```python
from build123d import *

# Parameters (mm, degrees)
BOSS_EXTRUDE1_DEPTH        = 1.5
SKETCH3_R                  = 2.5
SKETCH3_R_2                = 1
SKETCH3_R_3                = 2
BOSS_EXTRUDE2_DEPTH        = 3
F_4_8_4_8_DIAMETER_HOLE1_D = 4.8
SKETCH7_R                  = 4.75
SKETCH7_R_2                = 2.4
BOSS_EXTRUDE3_DEPTH        = 2.7
F_2_0MM_DOWEL_HOLE1_D      = 2
CHAMFER1_SIZE              = 1
SKETCH15_R                 = 2.38125
CUT_EXTRUDE1_DEPTH         = 126.335549626


with BuildPart() as part:
    # Sketch2 → Boss-Extrude1 (new, symmetric)
    with BuildSketch(Plane(origin=(0, 0, 0), x_dir=(1, 0, 0), z_dir=(0, 1, 0))):
        with BuildLine():
            Line((-50, -110), (50, -110))
            ThreePointArc((50, -110), (57.071067812, -107.071067812), (60, -100))
            Line((60, -100), (60, 100))
            ThreePointArc((60, 100), (57.071067812, 107.071067812), (50, 110))
            Line((50, 110), (-50, 110))
            ThreePointArc((-50, 110), (-57.071067812, 107.071067812), (-60, 100))
            Line((-60, 100), (-60, -100))
            ThreePointArc((-60, -100), (-57.071067812, -107.071067812), (-50, -110))
        make_face()
    extrude(amount=BOSS_EXTRUDE1_DEPTH, both=True)

    # Sketch3 → Boss-Extrude2 (add)
    # profile 1 of 16: a face of its own
    with BuildSketch(Plane(origin=(0, 1.5, 0), x_dir=(1, 0, 0), z_dir=(0, 1, 0))):
        with Locations(Location((41.24318761, -46.24391141, 0), (0, 0, 90))):
            Circle(SKETCH3_R)
        with Locations(Location((41.24318761, -46.24391141, 0), (0, 0, 270))):
            Circle(SKETCH3_R_2, mode=Mode.SUBTRACT)
    # profile 2 of 16: a face of its own
    with BuildSketch(Plane(origin=(0, 1.5, 0), x_dir=(1, 0, 0), z_dir=(0, 1, 0))):
        with Locations(Location((3.86368673, -46.24391141, 0), (0, 0, 90))):
            Circle(SKETCH3_R)
        with Locations(Location((3.86368673, -46.24391141, 0), (0, 0, 270))):
            Circle(SKETCH3_R_2, mode=Mode.SUBTRACT)
    # profile 3 of 16: a face of its own
    with BuildSketch(Plane(origin=(0, 1.5, 0), x_dir=(1, 0, 0), z_dir=(0, 1, 0))):
        with Locations(Location((3.86368673, -82.98571173, 0), (0, 0, 90))):
            Circle(SKETCH3_R)
        with Locations(Location((3.86368673, -82.98571173, 0), (0, 0, 270))):
            Circle(SKETCH3_R_2, mode=Mode.SUBTRACT)
    # profile 4 of 16: a face of its own
    with BuildSketch(Plane(origin=(0, 1.5, 0), x_dir=(1, 0, 0), z_dir=(0, 1, 0))):
        with Locations(Location((41.24318761, -82.98571173, 0), (0, 0, 90))):
            Circle(SKETCH3_R)
        with Locations(Location((41.24318761, -82.98571173, 0), (0, 0, 270))):
            Circle(SKETCH3_R_2, mode=Mode.SUBTRACT)
    # profile 5 of 16: a face of its own
    with BuildSketch(Plane(origin=(0, 1.5, 0), x_dir=(1, 0, 0), z_dir=(0, 1, 0))):
        with Locations(Location((-10.13631327, -24.98571173, 0), (0, 0, 90))):
            Circle(SKETCH3_R)
        with Locations(Location((-10.13631327, -24.98571173, 0), (0, 0, 270))):
            Circle(SKETCH3_R_2, mode=Mode.SUBTRACT)
    # profile 6 of 16: a face of its own
    with BuildSketch(Plane(origin=(0, 1.5, 0), x_dir=(1, 0, 0), z_dir=(0, 1, 0))):
        with Locations(Location((-10.13631327, 11.75608859, 0), (0, 0, 90))):
            Circle(SKETCH3_R)
        with Locations(Location((-10.13631327, 11.75608859, 0), (0, 0, 270))):
            Circle(SKETCH3_R_2, mode=Mode.SUBTRACT)
    # profile 7 of 16: a face of its own
    with BuildSketch(Plane(origin=(0, 1.5, 0), x_dir=(1, 0, 0), z_dir=(0, 1, 0))):
        with Locations(Location((27.24318761, 11.75608859, 0), (0, 0, 90))):
            Circle(SKETCH3_R)
        with Locations(Location((27.24318761, 11.75608859, 0), (0, 0, 270))):
            Circle(SKETCH3_R_2, mode=Mode.SUBTRACT)
    # profile 8 of 16: a face of its own
    with BuildSketch(Plane(origin=(0, 1.5, 0), x_dir=(1, 0, 0), z_dir=(0, 1, 0))):
        with Locations(Location((27.24318761, -24.98571173, 0), (0, 0, 90))):
            Circle(SKETCH3_R)
        with Locations(Location((27.24318761, -24.98571173, 0), (0, 0, 270))):
            Circle(SKETCH3_R_2, mode=Mode.SUBTRACT)
    # profile 9 of 16: a face of its own
    with BuildSketch(Plane(origin=(0, 1.5, 0), x_dir=(1, 0, 0), z_dir=(0, 1, 0))):
        with Locations(Location((-48.56, -75.45, 0), (0, 0, 90))):
            Circle(SKETCH3_R_3)
        with Locations(Location((-48.56, -75.45, 0), (0, 0, 270))):
            Circle(SKETCH3_R_2, mode=Mode.SUBTRACT)
    # profile 10 of 16: a face of its own
    with BuildSketch(Plane(origin=(0, 1.5, 0), x_dir=(1, 0, 0), z_dir=(0, 1, 0))):
        with Locations(Location((-32.54, -45.15, 0), (0, 0, 90))):
            Circle(SKETCH3_R_3)
        with Locations(Location((-32.54, -45.15, 0), (0, 0, 270))):
            Circle(SKETCH3_R_2, mode=Mode.SUBTRACT)
    # profile 11 of 16: a face of its own
    with BuildSketch(Plane(origin=(0, 1.5, 0), x_dir=(1, 0, 0), z_dir=(0, 1, 0))):
        with Locations(Location((-48.56, -21.95, 0), (0, 0, 90))):
            Circle(SKETCH3_R_3)
        with Locations(Location((-48.56, -21.95, 0), (0, 0, 270))):
            Circle(SKETCH3_R_2, mode=Mode.SUBTRACT)
    # profile 12 of 16: a face of its own
    with BuildSketch(Plane(origin=(0, 1.5, 0), x_dir=(1, 0, 0), z_dir=(0, 1, 0))):
        with Locations(Location((-32.54, 8.35, 0), (0, 0, 90))):
            Circle(SKETCH3_R_3)
        with Locations(Location((-32.54, 8.35, 0), (0, 0, 270))):
            Circle(SKETCH3_R_2, mode=Mode.SUBTRACT)
    # profile 13 of 16: a face of its own
    with BuildSketch(Plane(origin=(0, 1.5, 0), x_dir=(1, 0, 0), z_dir=(0, 1, 0))):
        with Locations(Location((-39.7, 32.2, 0), (0, 0, 90))):
            Circle(SKETCH3_R)
        with Locations(Location((-39.7, 32.2, 0), (0, 0, 270))):
            Circle(SKETCH3_R_2, mode=Mode.SUBTRACT)
    # profile 14 of 16: a face of its own
    with BuildSketch(Plane(origin=(0, 1.5, 0), x_dir=(1, 0, 0), z_dir=(0, 1, 0))):
        with Locations(Location((-38.6, 80, 0), (0, 0, 90))):
            Circle(SKETCH3_R)
        with Locations(Location((-38.6, 80, 0), (0, 0, 270))):
            Circle(SKETCH3_R_2, mode=Mode.SUBTRACT)
    # profile 15 of 16: a face of its own
    with BuildSketch(Plane(origin=(0, 1.5, 0), x_dir=(1, 0, 0), z_dir=(0, 1, 0))):
        with Locations(Location((12.2, 36.9, 0), (0, 0, 90))):
            Circle(SKETCH3_R)
        with Locations(Location((12.2, 36.9, 0), (0, 0, 270))):
            Circle(SKETCH3_R_2, mode=Mode.SUBTRACT)
    # profile 16 of 16: a face of its own
    with BuildSketch(Plane(origin=(0, 1.5, 0), x_dir=(1, 0, 0), z_dir=(0, 1, 0))):
        with Locations(Location((12.2, 64.8, 0), (0, 0, 90))):
            Circle(SKETCH3_R)
        with Locations(Location((12.2, 64.8, 0), (0, 0, 270))):
            Circle(SKETCH3_R_2, mode=Mode.SUBTRACT)
    extrude(amount=BOSS_EXTRUDE2_DEPTH)

    # Ø4.8 (4.8) Diameter Hole1 (through all)
    with Locations(Plane(origin=(0, 1.5, 0), x_dir=(1, 0, 0), z_dir=(0, 1, 0))):
        with Locations((51, 101), (51, -101), (-51, -101), (-51, 101)):
            Hole(F_4_8_4_8_DIAMETER_HOLE1_D / 2)

    # Sketch7 → Boss-Extrude3 (add)
    # profile 1 of 4: a face of its own
    with BuildSketch(Plane(origin=(0, 1.5, 0), x_dir=(1, 0, 0), z_dir=(0, 1, 0))):
        with Locations(Location((51, 101, 0), (0, 0, 90))):
            Circle(SKETCH7_R)
        with Locations(Location((51, 101, 0), (0, 0, 270))):
            Circle(SKETCH7_R_2, mode=Mode.SUBTRACT)
    # profile 2 of 4: a face of its own
    with BuildSketch(Plane(origin=(0, 1.5, 0), x_dir=(1, 0, 0), z_dir=(0, 1, 0))):
        with Locations(Location((-51, 101, 0), (0, 0, 90))):
            Circle(SKETCH7_R)
        with Locations(Location((-51, 101, 0), (0, 0, 270))):
            Circle(SKETCH7_R_2, mode=Mode.SUBTRACT)
    # profile 3 of 4: a face of its own
    with BuildSketch(Plane(origin=(0, 1.5, 0), x_dir=(1, 0, 0), z_dir=(0, 1, 0))):
        with Locations(Location((-51, -101, 0), (0, 0, 90))):
            Circle(SKETCH7_R)
        with Locations(Location((-51, -101, 0), (0, 0, 270))):
            Circle(SKETCH7_R_2, mode=Mode.SUBTRACT)
    # profile 4 of 4: a face of its own
    with BuildSketch(Plane(origin=(0, 1.5, 0), x_dir=(1, 0, 0), z_dir=(0, 1, 0))):
        with Locations(Location((51, -101, 0), (0, 0, 90))):
            Circle(SKETCH7_R)
        with Locations(Location((51, -101, 0), (0, 0, 270))):
            Circle(SKETCH7_R_2, mode=Mode.SUBTRACT)
    extrude(amount=BOSS_EXTRUDE3_DEPTH)

    # Ø2.0mm Dowel Hole1 (through all)
    with Locations(Plane(origin=(0, 1.5, 0), x_dir=(1, 0, 0), z_dir=(0, 1, 0))):
        with Locations((27.24318761, -24.98571173), (27.24318761, 11.75608859), (-10.13631327, -24.98571173), (-10.13631327, 11.75608859), (3.86368673, -46.24391141), (41.24318761, -46.24391141), (41.24318761, -82.98571173), (3.86368673, -82.98571173), (12.2, 36.9), (12.2, 64.8), (-38.6, 80), (-39.7, 32.2), (-32.54, 8.35), (-48.56, -21.95), (-48.56, -75.45), (-32.54, -45.15), (34.8, 38), (34.8, 32)):
            Hole(F_2_0MM_DOWEL_HOLE1_D / 2)

    # Chamfer1
    chamfer1_edges = [part.edges().sort_by_distance(p)[0] for p in [
        (-38.6, 1.5, -77.5),
        (12.2, 1.5, -34.4),
        (12.2, 1.5, -62.3),
        (51, 1.5, -96.25),
        (-51, 1.5, -96.25),
        (-51, 1.5, 105.75),
        (51, 1.5, 105.75),
        (41.24318761, 1.5, 48.74391141),
        (3.86368673, 1.5, 48.74391141),
        (3.86368673, 1.5, 85.48571173),
        (41.24318761, 1.5, 85.48571173),
        (-10.13631327, 1.5, 27.48571173),
        (-10.13631327, 1.5, -9.25608859),
        (27.24318761, 1.5, -9.25608859),
        (27.24318761, 1.5, 27.48571173),
        (-48.56, 1.5, 77.45),
        (-32.54, 1.5, 47.15),
        (-48.56, 1.5, 23.95),
        (-32.54, 1.5, -6.35),
        (-39.7, 1.5, -29.7),
    ]]
    chamfer(chamfer1_edges, length=CHAMFER1_SIZE)

    # Sketch15 → Cut-Extrude1 (cut, through all)
    with BuildSketch(Plane(origin=(0, 1.5, 0), x_dir=(1, 0, 0), z_dir=(0, 1, 0))):
        with Locations(Location((-4, -60.3, 0), (0, 0, 270))):
            Circle(SKETCH15_R)
        with Locations(Location((-25, -60.3, 0), (0, 0, 270))):
            Circle(SKETCH15_R)
    extrude(amount=-CUT_EXTRUDE1_DEPTH, mode=Mode.SUBTRACT)


solid = part.part
```
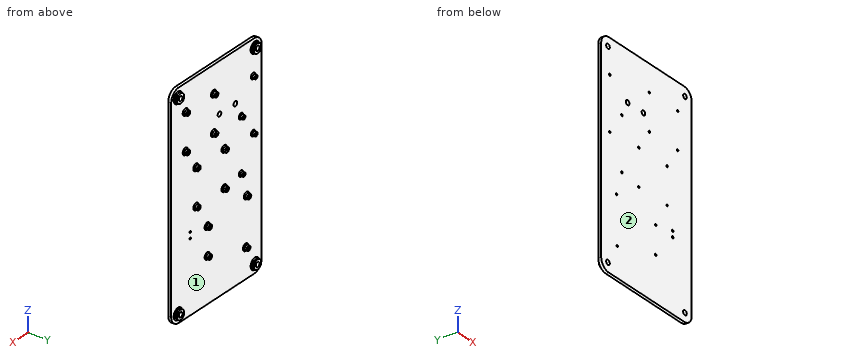
Read the model definition and answer for the solid it produces. Units are mm, in the model's axes. Face numbers are marked on the shaded views. Coordinates: 2 decimals unless noted, no trailing zeros. Write each loop counter-clockwise with the first axis right and the second up, starting at its lowest first coordinate (ties: lowest second). Pieces come first, ordered by that corner, then holes. Notation, with made-up numbers: (-32.75, 74.25) - (23.25, 74.25) arc R16 ccw to (23.25, 83.25) - close; hole circle Ø3 at (-2.5, -21.5). An arc over 180 degrees is marked (long way). Answer as a JSON object with one key per item and string values. Group by question number.
1. Each of these flat-tipped pins is pushed along its axis until it touches: P1, Ø1, axis at x = 5, y = 2.5, coming from the -Z side (3 decimals); P2, Ø7.5, axis at x = 51, z = -101, coming from the +Y side. Where does it stop, or does it pass through?
2. A cutting plane is placed at A-A (z = 90). Determine the outline of the cut face in (x, y), plus the area to 3 significant figures.
3. Consider L1, parallel to Z at x = 12.2, y = -0.4; L2, parallel to Z at x = -33, y = 3.85; L3, parallel to Z at x = -32.54, y = 2.2. Determine where each line is inside the solid, lowest interval first. Write a range as [from, to].
4. The mould has two halves that part along Z. Classify the marked faces 1 and 2: +Z half, -Z half, draft (parallel to the pull), parting line (faces both ways), or undercut.
Worked out:
{
 "1": {"P1": "stops at z = 43.435", "P2": "stops at y = 4.2"},
 "2": {"outline": "(-60, -1.5) - (60, -1.5) - (60, 1.5) - (-60, 1.5) - close", "area": "360 mm²"},
 "3": {"L1": "z = [-110, -65.8], [-63.8, -37.9], [-35.9, 110]", "L2": "z = [-10.3, -9.24], [-7.46, -6.4], [43.2, 44.26], [46.04, 47.1]", "L3": "z = [-10.65, -9.35], [-7.35, -6.05], [42.85, 44.15], [46.15, 47.45]"},
 "4": {"face 1": "undercut", "face 2": "draft"}
}
